Design review of the part built by this model. Coordinates are the model's own, in mm. A direction names the side the tool comes from. Give positions to 0.01 mm unless a question says otherwise; leave off trailing zeros. Loops run counter-clockwise (first coordinate to the right, second up) from the corner with the lowest first, then second, coordinate; pieces in that order, holes last. Notation, with made-up numbers: M 45,73 L 54,73 A20 ccw 54,84 Z; hole C 89.5,73 d2. An arc over 180 degrees is marked long. Use CSV: the item, a comma, the result in double quotes.
from build123d import *

# Parameters (mm, degrees)
SKETCH1_R           = 1.650000007
BOSS_EXTRUDE1_DEPTH = 3.5
SKETCH8_R           = 5
CUT_EXTRUDE3_DEPTH  = 10
SKETCH9_R           = 1.6
CUT_EXTRUDE4_DEPTH  = 10
BOSS_EXTRUDE5_DEPTH = 30
FILLET4_R           = 2
SKETCH13_R          = 9.5
BOSS_EXTRUDE6_DEPTH = 30
FILLET5_R           = 1
REVOLVE2_ANGLE      = 180


with BuildPart() as part:
    # Sketch1 → Boss-Extrude1 (new, symmetric)
    with BuildSketch(Plane(origin=(0, 0, 0), x_dir=(1, 0, 0), z_dir=(0, 1, 0))):
        with BuildLine():
            Line((-3.163944782, -93.076388076), (-20.805834618, -116.891940565))
            ThreePointArc((-20.805834618, -116.891940565), (-21.362478255, -119.119545961), (-20.180929864, -121.088307332))
            Line((-20.180929864, -121.088307332), (-6.520660553, -131.207449705))
            ThreePointArc((-6.520660553, -131.207449705), (-4.293055157, -131.764093342), (-2.324293786, -130.582544951))
            Line((-2.324293786, -130.582544951), (15.317595998, -106.766992534))
            ThreePointArc((15.317595998, -106.766992534), (16.298016652, -105.915587831), (17.546382486, -105.558240139))
            ThreePointArc((17.546382486, -105.558240139), (18.880171652, -105.241928098), (20.028844772, -104.493865997))
            Line((20.028844772, -104.493865997), (31.933718152, -88.422960925))
            ThreePointArc((31.933718152, -88.422960925), (32.812947077, -83.759740105), (28.619624318, -81.538318002))
            Line((28.619624318, -81.538318002), (0.643845867, -85.704349694))
            ThreePointArc((0.643845867, -85.704349694), (-2.081865152, -87.422063847), (-2.657041002, -90.592113564))
            ThreePointArc((-2.657041002, -90.592113564), (-2.635147269, -91.890433717), (-3.163944782, -93.076388076))
        make_face()
        with Locations(Location((1.233011719, -89.660722224, 0), (0, 0, 90))):
            Circle(SKETCH1_R, mode=Mode.SUBTRACT)
        with Locations(Location((29.20879017, -85.494690532, 0), (0, 0, 90))):
            Circle(SKETCH1_R, mode=Mode.SUBTRACT)
        with Locations(Location((17.30391679, -101.565595604, 0), (0, 0, 90))):
            Circle(SKETCH1_R, mode=Mode.SUBTRACT)
    extrude(amount=BOSS_EXTRUDE1_DEPTH, both=True)

    # Sketch8 → Cut-Extrude3 (cut)
    with BuildSketch(Plane(origin=(0, 3.5, 0), x_dir=(1, 0, 0), z_dir=(0, 1, 0))):
        with Locations((27.647963735, -94.208486751)):
            Circle(SKETCH8_R)
    extrude(amount=-CUT_EXTRUDE3_DEPTH, mode=Mode.SUBTRACT)

    # Sketch9 → Cut-Extrude4 (cut)
    with BuildSketch(Plane(origin=(0, 3.5, 0), x_dir=(1, 0, 0), z_dir=(0, 1, 0))):
        with Locations(Location((-6.267193351, -106.505511433, 0), (0, 0, 270))):
            Circle(SKETCH9_R)
        with Locations(Location((3.375349692, -113.648435461, 0), (0, 0, 270))):
            Circle(SKETCH9_R)
        with Locations(Location((-4.958061673, -124.898069011, 0), (0, 0, 270))):
            Circle(SKETCH9_R)
        with Locations(Location((-14.600604716, -117.755144983, 0), (0, 0, 270))):
            Circle(SKETCH9_R)
    extrude(amount=-CUT_EXTRUDE4_DEPTH, mode=Mode.SUBTRACT)

    # Sketch11 → Boss-Extrude5 (add)
    with BuildSketch(Plane.XZ.offset(3.5)):
        with BuildLine():
            Line((-3.514107133, 98.589040232), (10.146162178, 108.708182605))
            ThreePointArc((10.146162178, 108.708182605), (11.327710569, 110.676943976), (10.771066932, 112.904549372))
            Line((10.771066932, 112.904549372), (-2.324293786, 130.582544951))
            ThreePointArc((-2.324293786, 130.582544951), (-4.293055157, 131.764093342), (-6.520660553, 131.207449705))
            Line((-6.520660553, 131.207449705), (-20.180929864, 121.088307332))
            ThreePointArc((-20.180929864, 121.088307332), (-21.362478255, 119.119545961), (-20.805834618, 116.891940565))
            Line((-20.805834618, 116.891940565), (-7.710473901, 99.213944986))
            ThreePointArc((-7.710473901, 99.213944986), (-5.741712529, 98.032396595), (-3.514107133, 98.589040232))
        make_face()
    extrude(amount=BOSS_EXTRUDE5_DEPTH)

    # Fillet4
    fillet4_edges = [part.edges().sort_by_distance(p)[0] for p in [
        (-21.362478255, -33.5, 119.119545961),
        (-14.258154259, -33.5, 108.052942775),
        (-5.741712529, -33.5, 98.032396595),
        (3.316027522, -33.5, 103.648611418),
        (11.327710569, -33.5, 110.676943976),
        (4.223386573, -33.5, 121.743547162),
        (-4.293055157, -33.5, 131.764093342),
        (-13.350795209, -33.5, 126.147878519),
    ]]
    fillet(fillet4_edges, radius=FILLET4_R)

    # Sketch13 → Boss-Extrude6 (add)
    with BuildSketch(Plane.XZ.offset(33.5)):
        with Locations(Location((-5.017383843, 114.898244969, 0), (0, 0, 36.530004657))):
            Circle(SKETCH13_R)
    extrude(amount=BOSS_EXTRUDE6_DEPTH)

    # Fillet5
    fillet5_edges = [part.edges().sort_by_distance(p)[0] for p in [
        (-10.672198638, -33.5, 122.531924922),
        (0.637430952, -33.5, 107.264565015),
    ]]
    fillet(fillet5_edges, radius=FILLET5_R)

    # Sketch14 → Revolve2 (revolve)
    with BuildSketch(Plane.XZ.offset(63.5)):
        with BuildLine():
            Line((-5.017383843, 124.398244969), (-5.017383843, 105.398244968))
            ThreePointArc((-5.017383843, 105.398244968), (4.482616157, 114.898244969), (-5.017383843, 124.398244969))
        make_face()
    revolve(axis=Axis((-5.017383843, -63.5, 124.398244969), (0, 0, -1)), revolution_arc=REVOLVE2_ANGLE)


solid = part.part
(1) We need section B-B on y = -62.5. State the section outline as (x, z) points, then the cut area to 3 significant figures.
A:
outline,"C -5.02,114.9 d19"
area,"284 mm²"
(2) Clearance check with flat-ended pins moving along their axes: P1, Ø1, axis at x = 4, z = 113.5, coming from the +Y side; P2, Ø4, axis at x = 29.21, z = 85.49, coming from the -Y side; P3, Ø5, axis at x = 3.38, z = 113.65, coming from the -Y side. State where each tip first meets the part, or that it passes through.
A:
P1,"y = -3.5"
P2,"y = -3.5"
P3,"y = -70.87"
(3) Wall thickness on line 1 along Y through (x, z) = (18.5, 95); line 2 along X through (y, z) = (-2.5, 124); line 3 along Y through (x, z) = (6, 112): over which ranges is each line inside the solid? List them lowest first. Write a range as [from, to].
A:
line 1,"[-3.5, 3.5]"
line 2,"[-16.25, -6.28], [-3.63, 2.55]"
line 3,"[-33.5, 3.5]"
(4) Machinability: for faces 5 (the flat face through (-13.255, -13.755, 126.219)), 6 (the cylindrical face through (11.32, -17.3, 110.64)), 7 (the cylindrical face through (-5.774, -17.304, 98.037)), 8 (the cylindrical face through (3.45, 0.05, 112.05)), which of the approach directions +Z, -Z, +X, -X, +Y, -Y give a long, thin tool a straight path to every point of the face, cutting with its end or side? Answer none if there is none.
A:
face 5,"+Z, -X, +Y, -Y"
face 6,"+X, -Y"
face 7,"-Z, -Y"
face 8,"+Y"
(5) We need section A-A on y = -26.5. State the section outline as (x, z) points, then the cut area to 3 significant figures.
A:
outline,"M -20.81,116.89 L -7.71,99.21 A3 ccw -3.51,98.59 L 10.15,108.71 A3 ccw 10.77,112.9 L -2.32,130.58 A3 ccw -6.52,131.21 L -20.18,121.09 A3 ccw Z"
area,"636 mm²"
(6) We need section C-C on x = 14. State the section outline as (y, z) points.
A:
outline,"M -3.5,83.72 L 3.5,83.72 L 3.5,108.55 L -3.5,108.55 Z"
(7) The part is to be moulded in two halves that separate along X. For faces 1 (the cylindrical face through (0.57, -48.69, 122.58)), 2 (the cylindrical face through (-13.683, -32.93, 108.287)), 3 (the flat face through (-6, -3.5, 107)), 4 (the flat face through (1, -33.5, 106)), say which applies: released by +X, released by -X, zero draft, split by the parting line, or undercut.
A:
face 1,"split by the parting line"
face 2,"released by -X"
face 3,"undercut"
face 4,"zero draft"
